```python
from build123d import *

# Parameters (mm, degrees)
SKETCH_2_W           = 65.2997206
SKETCH_2_H           = 38
SKETCH_2_R           = 1.00000254
SKETCH_2_R_2         = 0.922218434
SKETCH_2_R_3         = 1.5
EXTRUDE_2_DEPTH      = 4.5
SKETCH_3_R           = 1.5
CUT_EXTRUDE_2_DEPTH  = 2.5
SKETCH_5_W           = 65.2997206
SKETCH_5_H           = 38
SKETCH_5_W_2         = 61.2997206
SKETCH_5_H_2         = 34
EXTRUDE_3_DEPTH      = 21
EXTRUDE_3_DEPTH_BACK = 16
SKETCH_7_W           = 8.214112973
SKETCH_7_H           = 3.795011114
CUT_EXTRUDE_4_DEPTH  = 3
SKETCH_8_W           = 4
SKETCH_8_H           = 9.575559499
CUT_EXTRUDE_5_DEPTH  = 3
SKETCH_9_W           = 9.326303795
SKETCH_9_H           = 4.202278939
CUT_EXTRUDE_6_DEPTH  = 3
CUT_EXTRUDE_7_DEPTH  = 10
SKETCH_15_R          = 1.75
CUT_EXTRUDE_8_DEPTH  = 1.5
SKETCH_18_W          = 61.2997206
SKETCH_18_H          = 35
CUT_EXTRUDE_9_DEPTH  = 2
SKETCH_19_W          = 1.5
SKETCH_19_H          = 4
CUT_EXTRUDE_10_DEPTH = 2


with BuildPart() as part:
    # 草图2 → 凸台-拉伸2 (new body)
    with BuildSketch(Plane(origin=(0, 0, -6), x_dir=(-1, 0, 0), z_dir=(0, 0, -1))):
        with Locations((29.273558547, -24.066548133)):
            Rectangle(SKETCH_2_W, SKETCH_2_H)
        with Locations((1.016002032, -11.24978156)):
            Circle(SKETCH_2_R, mode=Mode.SUBTRACT)
        with Locations((0.889001778, -36.83007366)):
            Circle(SKETCH_2_R, mode=Mode.SUBTRACT)
        with Locations((57.658115316, -36.64983236)):
            Circle(SKETCH_2_R, mode=Mode.SUBTRACT)
        with Locations((57.658115316, -11.24978156)):
            Circle(SKETCH_2_R_2, mode=Mode.SUBTRACT)
        with Locations((29.273558547, -32.316548133)):
            Circle(SKETCH_2_R_3, mode=Mode.SUBTRACT)
        with BuildLine():
            Line((27.785407033, -15.816548133), (27.785407033, -13.183619987))
            ThreePointArc((27.785407033, -13.183619987), (29.273558547, -11.695468472), (30.761710061, -13.183619987))
            Line((30.761710061, -13.183619987), (30.761710061, -15.816548133))
            ThreePointArc((30.761710061, -15.816548133), (29.273558547, -17.304699647), (27.785407033, -15.816548133))
        make_face(mode=Mode.SUBTRACT)
    extrude(amount=EXTRUDE_2_DEPTH)

    # 草图3 → 切除-拉伸2 (cut)
    with BuildSketch(Plane(origin=(0, 0, -6), x_dir=(-1, 0, 0), z_dir=(0, 0, -1))):
        Polygon((29.273558547, -18.991974614), (32.023558547, -17.404261373), (32.023558547, -14.920341582), (32.023558547, -14.228834893), (32.023558547, -11.744915102), (29.273558547, -10.157201862), (26.523558547, -11.744915102), (26.523558547, -14.228834893), (26.523558547, -14.920341582), (26.523558547, -17.404261373), align=None)
        with BuildLine():
            ThreePointArc((30.761710061, -15.816548133), (29.273558547, -17.304699647), (27.785407033, -15.816548133))
            Line((27.785407033, -15.816548133), (27.785407033, -13.183619987))
            ThreePointArc((27.785407033, -13.183619987), (29.273558547, -11.695468472), (30.761710061, -13.183619987))
            Line((30.761710061, -13.183619987), (30.761710061, -15.816548133))
        make_face(mode=Mode.SUBTRACT)
        Polygon((26.523558547, -30.728834893), (26.523558547, -33.904261373), (29.273558547, -35.491974614), (32.023558547, -33.904261373), (32.023558547, -30.728834893), (29.273558547, -29.141121653), align=None)
        with Locations((29.273558547, -32.316548133)):
            Circle(SKETCH_3_R, mode=Mode.SUBTRACT)
    extrude(amount=CUT_EXTRUDE_2_DEPTH, mode=Mode.SUBTRACT)

    # 草图5 → 凸台-拉伸3 (add, two sides)
    with BuildSketch(Plane(origin=(0, 0, -10.5), x_dir=(-1, 0, 0), z_dir=(0, 0, -1))) as extrude_3_sk:
        with Locations((29.273558547, -24.066548133)):
            Rectangle(SKETCH_5_W, SKETCH_5_H)
        with Locations((29.273558547, -24.066548133)):
            Rectangle(SKETCH_5_W_2, SKETCH_5_H_2, mode=Mode.SUBTRACT)
    extrude(amount=EXTRUDE_3_DEPTH)
    extrude(extrude_3_sk.sketch, amount=-EXTRUDE_3_DEPTH_BACK)

    # 草图7 → 切除-拉伸4 (cut)
    with BuildSketch(Plane(origin=(0, -5.066548133, 0), x_dir=(1, 0, 0), z_dir=(0, 1, 0))):
        with Locations((-50.955145133, -3.662545243)):
            Rectangle(SKETCH_7_W, SKETCH_7_H)
    extrude(amount=-CUT_EXTRUDE_4_DEPTH, mode=Mode.SUBTRACT)

    # 草图8 → 切除-拉伸5 (cut)
    with BuildSketch(Plane.ZY.offset(61.923418847)):
        with Locations((3.6000508, -23.483057223)):
            Rectangle(SKETCH_8_W, SKETCH_8_H)
    extrude(amount=-CUT_EXTRUDE_5_DEPTH, mode=Mode.SUBTRACT)

    # 草图9 → 切除-拉伸6 (cut)
    with BuildSketch(Plane.XZ.offset(43.066548133)):
        with Locations((-44.464129124, 3.49891133)):
            Rectangle(SKETCH_9_W, SKETCH_9_H)
    extrude(amount=-CUT_EXTRUDE_6_DEPTH, mode=Mode.SUBTRACT)

    # 草图13 → 切除-拉伸7 (cut)
    with BuildSketch(Plane.XY.offset(-6)):
        Polygon((-59.923418847, -16.066514367), (-59.923418847, -19.252115931), (-54.525349934, -19.252115931), (-54.525349934, -41.066548133), (-34.525349934, -41.066548133), (-34.525349934, -7.066548133), (-54.525349934, -7.066548133), (-54.525349934, -12.880912803), (-54.525349934, -16.066514367), align=None)
    extrude(amount=-CUT_EXTRUDE_7_DEPTH, mode=Mode.SUBTRACT)

    # 草图15 → 切除-拉伸8 (cut)
    with BuildSketch(Plane(origin=(0, 0, -10.5), x_dir=(-1, 0, 0), z_dir=(0, 0, -1))):
        with Locations((1.016002032, -11.24978156)):
            Circle(SKETCH_15_R)
        with Locations((57.658115316, -11.24978156)):
            Circle(SKETCH_15_R)
        with Locations((0.889001778, -36.83007366)):
            Circle(SKETCH_15_R)
        with Locations((57.658115316, -36.64983236)):
            Circle(SKETCH_15_R)
    extrude(amount=-CUT_EXTRUDE_8_DEPTH, mode=Mode.SUBTRACT)

    # 草图18 → 切除-拉伸9 (cut)
    with BuildSketch(Plane(origin=(0, 0, -31.5), x_dir=(-1, 0, 0), z_dir=(0, 0, -1))):
        with Locations((29.273558547, -24.066548133)):
            Rectangle(SKETCH_18_W, SKETCH_18_H)
    extrude(amount=-CUT_EXTRUDE_9_DEPTH, mode=Mode.SUBTRACT)

    # 草图19 → 切除-拉伸10 (cut)
    with BuildSketch(Plane.ZY.offset(-1.376301753)):
        with Locations((-28.75, -9.066548133)):
            Rectangle(SKETCH_19_W, SKETCH_19_H)
        with Locations((-28.75, -39.066548133)):
            Rectangle(SKETCH_19_W, SKETCH_19_H)
    extrude(amount=-CUT_EXTRUDE_10_DEPTH, mode=Mode.SUBTRACT)


solid = part.part
```
Can you work these out from the model? Positions are in its coordinate system, mm. A direction names the side the tool comes from. Coordinates: 2 decimals unless noted, no trailing zeros. Loops run counter-clockwise (first coordinate to the right, second up) from the corner with the lowest first, then second, coordinate; pieces in that order, holes last. Notation, with made-up numbers: (53.5, 32) -> (63.5, 32) arc R33 ccw to (63.5, 69) -> close; hole circle Ø9 at (61.25, -30.5). An arc over 180 degrees is marked (long way). Answer as a JSON object with one key per item and string values.
1) Thinking about a two-plate mould opening in Y: for faces 1 (the face through (-0.76, -35.84, -7.48)), 2 (the face through (-29, -43.067, -13)), 3 (the face through (-60.2, -38.4, 5.5)), which applies, pulls with the +Y half, pulls with the -Y half, needs draft (parallel to the pull), parting line crosses it, or undercut?
Results:
{"face 1": "undercut", "face 2": "pulls with the -Y half", "face 3": "needs draft"}
2) Imagine slicing it at D-D (y = -26). Please give me the cut outline in (x, z).
Results:
{"outline": "(-61.92, -31.5) -> (-59.92, -31.5) -> (-59.92, -10.5) -> (-54.53, -10.5) -> (-54.53, -6) -> (-59.92, -6) -> (-59.92, 1.6) -> (-61.92, 1.6) -> close; (-34.53, -10.5) -> (1.38, -10.5) -> (1.38, -31.5) -> (3.38, -31.5) -> (3.38, 5.5) -> (1.38, 5.5) -> (1.38, -6) -> (-34.53, -6) -> close"}
3) Imagine slicing it at A-A (x = -44.5). Please give me the cut outline in (y, z).
Results:
{"outline": "(-43.07, -31.5) -> (-41.57, -31.5) -> (-41.57, -29.5) -> (-41.07, -29.5) -> (-41.07, 1.4) -> (-43.07, 1.4) -> close; (-7.07, -29.5) -> (-6.57, -29.5) -> (-6.57, -31.5) -> (-5.07, -31.5) -> (-5.07, 5.5) -> (-7.07, 5.5) -> close"}
4) For P1, Ø4, axis at x = -19, y = -23, coming from the -Z side; P2, Ø6, axis at x = -28, y = -33, coming from the +Z side; P3, Ø1, axis at x = -0.5, y = -11.5, coming from the -Z side, each with a flat end and sliding along its axis, tell me the tip position at first contact or that it passes through.
Results:
{"P1": "stops at z = -10.5", "P2": "stops at z = -6", "P3": "stops at z = -9"}
5) Imagine slicing it at B-B (y = -14). Please give me the cut outline in (x, z).
Results:
{"outline": "(-61.92, -31.5) -> (-59.92, -31.5) -> (-59.92, -10.5) -> (-54.53, -10.5) -> (-54.53, -6) -> (-59.92, -6) -> (-59.92, 5.5) -> (-61.92, 5.5) -> close; (-34.53, -10.5) -> (-30.76, -10.5) -> (-30.76, -8.5) -> (-32.02, -8.5) -> (-32.02, -6) -> (-34.53, -6) -> close; (-27.79, -10.5) -> (1.38, -10.5) -> (1.38, -31.5) -> (3.38, -31.5) -> (3.38, 5.5) -> (1.38, 5.5) -> (1.38, -6) -> (-26.52, -6) -> (-26.52, -8.5) -> (-27.79, -8.5) -> close"}
6) For faces 4 (the face through (-55.062, -6, 4)), 5 (the face through (-27.785, -15, -9)), 6 (the face through (-26.524, -15, -7)), 7 (the face through (-59, -37, -9)), which set-ups out of +Z, -Z, +X, -X, +Y, -Y let a thin tool reach every point of the face, with its end or its side?
Results:
{"face 4": "+Z, +Y", "face 5": "+Z, -Z", "face 6": "+Z", "face 7": "-Z"}
7) If I drill on line 1 (X direction, y = -25.5, z = 1); line 2 (Y direction, x = -22, z = -14); line 3 (Z direction, x = -25, y = -29), over which ranges is the centre line in solid material (lowest first)?
Results:
{"line 1": "x = -61.92 to -59.92, 1.38 to 3.38", "line 2": "y = -43.07 to -41.07, -7.07 to -5.07", "line 3": "z = -10.5 to -6"}
8) Imagine slicing it at C-C (z = 0). Please give me the cut outline in (x, y), then the cut area to 3 significant figures.
Results:
{"outline": "(-61.92, -43.07) -> (3.38, -43.07) -> (3.38, -5.07) -> (-61.92, -5.07) -> close; hole (-59.92, -41.07) -> (1.38, -41.07) -> (1.38, -7.07) -> (-59.92, -7.07) -> close", "area": "397 mm^2"}
